Can you work these out from the drawing? Everything is in mm from the part's minimum corner. A direction names the side the tool comes from. Give positions to 0.01 mm unless a question says otherwise; leave off trailing zeros. Write each loop counter-clockwise with the first axis right and the second up, starting at its lowest first coordinate (ties: lowest second). Pieces come first, ordered by that corner, then holes. Notation, with made-up numbers: (66.25, 69) -> (123.25, 69) arc R25 ccw to (123.25, 104) -> close; hole circle Ø10 at (-28.5, -14.75). An arc over 180 degrees is marked (long way). Use one line per item in the form item = value.
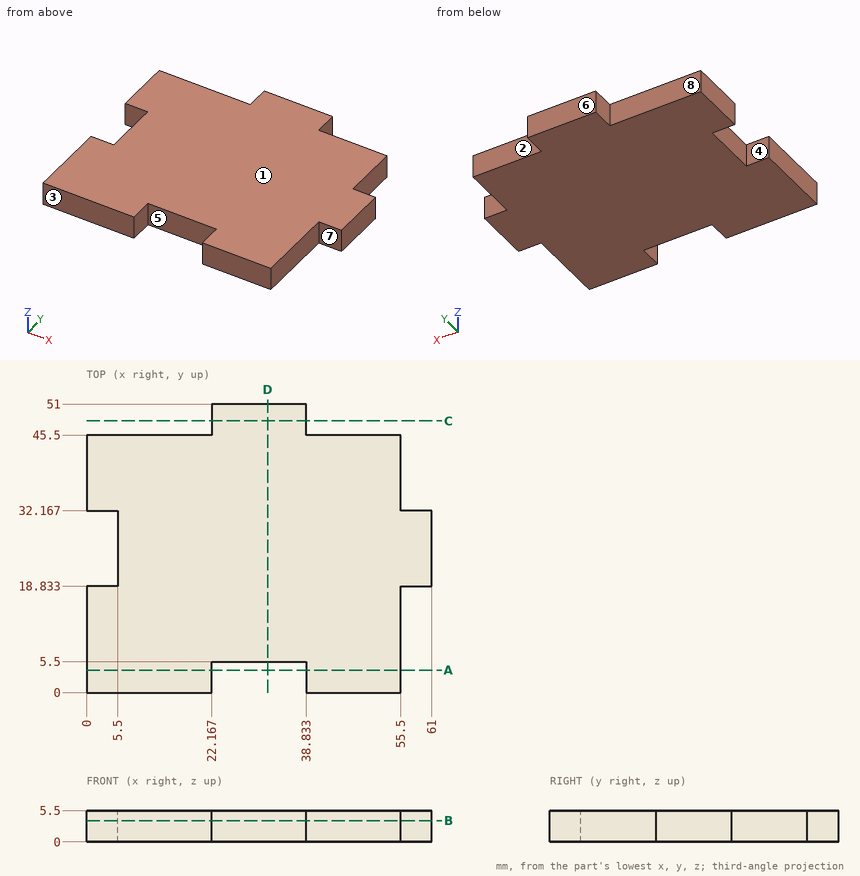
Q1. I want a section at A-A, the plane y = 4. Write out the boundary of the cut face in (x, z).
Result set:
outline = (0, 0) -> (22.17, 0) -> (22.17, 5.5) -> (0, 5.5) -> close; (38.83, 0) -> (55.5, 0) -> (55.5, 5.5) -> (38.83, 5.5) -> close
Q2. I want a section at C-C, the plane y = 48. Write out the boundary of the cut face in (x, z).
Result set:
outline = (22.17, 0) -> (38.83, 0) -> (38.83, 5.5) -> (22.17, 5.5) -> close
Q3. Will these pins go through, and if not, where does the flat tip stop? pin 1 Ø1.6 at (y, z) = (49.5, 3.5) entering from -X; pin 2 Ø3 at (x, z) = (31, 1.5) entering from -Y; pin 3 Ø1.6 at (x, z) = (59.5, 2) entering from +Y.
Result set:
pin_1 = 22.17
pin_2 = 5.5
pin_3 = 32.17
Q4. If we mould it in two halves opening along Y, with no side actions, what happens to the marked faces 1, 2, 3 and 4? For each: +Y half, -Y half, draft (parallel to the pull), parting line (faces both ways), or undercut.
Result set:
face_1 = draft
face_2 = +Y half
face_3 = -Y half
face_4 = undercut
Q5. I want a section at B-B, the plane z = 3.75. Write out the boundary of the cut face in (x, y).
Result set:
outline = (0, 0) -> (22.17, 0) -> (22.17, 5.5) -> (38.83, 5.5) -> (38.83, 0) -> (55.5, 0) -> (55.5, 18.83) -> (61, 18.83) -> (61, 32.17) -> (55.5, 32.17) -> (55.5, 45.5) -> (38.83, 45.5) -> (38.83, 51) -> (22.17, 51) -> (22.17, 45.5) -> (0, 45.5) -> (0, 32.17) -> (5.5, 32.17) -> (5.5, 18.83) -> (0, 18.83) -> close
Q6. I want a section at D-D, the plane x = 32. Write out the boundary of the cut face in (y, z), and give its area (3 significant figures).
Result set:
outline = (5.5, 0) -> (51, 0) -> (51, 5.5) -> (5.5, 5.5) -> close
area = 250 mm2
Q7. Which directions (+Z, -Z, +X, -X, +Y, -Y) give clear straight access to the entire face, cutting with the end or side of a thin tool? Please do the marked faces 5, 6, 7 and 8.
Result set:
face_5 = +Z, -Z, -Y
face_6 = +Z, -Z, +X, -X, +Y
face_7 = +Z, -Z, +X, -Y
face_8 = +Z, -Z, -X, +Y
Q8. If I drill on line 1 along X through (y, z) = (4.5, 0.9); line 2 along X through (y, z) = (33.5, 5); line 3 along Y through (x, z) = (46, 2.9), over which ranges is the centre line in solid material (lowest first)? Write a range as from..to.
Result set:
line_1 = 0..22.17, 38.83..55.5
line_2 = 0..55.5
line_3 = 0..45.5
